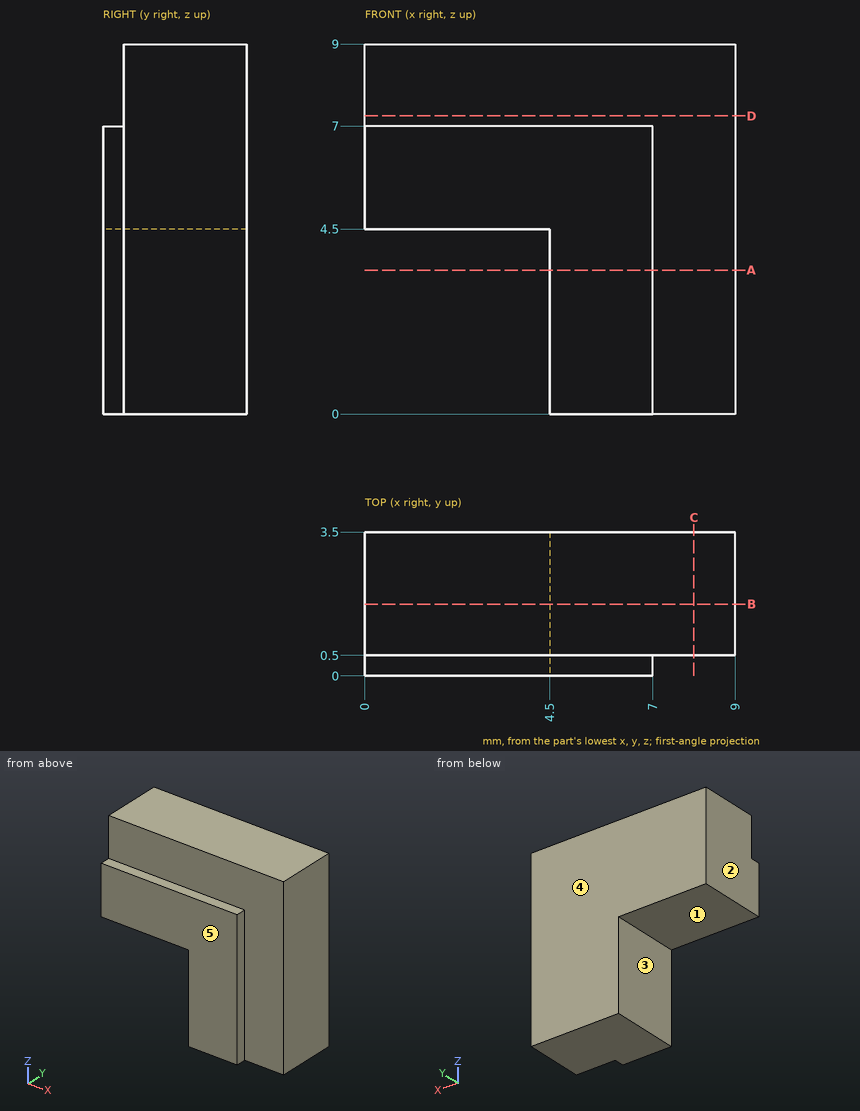
Design review of the part shown in the three views and the two pictorial views. Dimensions are in mm from the part's minimum x, y and z. A direction names the side the tool comes from. Give positions to 0.01 mm unless a question says otherwise; leave off trailing zeros. Write each loop counter-clockwise with the first axis right and the second up, starting at its lowest first coordinate (ties: lowest second). Pieces come first, ordered by that corner, then holes. Notation, with made-up numbers: M 72.5,31.5 L 85.5,31.5 A3 cw 85.5,36.5 Z; hole C 40.5,83.25 d10. An arc over 180 degrees is marked long. One line per question, with ' | ' between items. Start each with the question number.
Item 1: Wall thickness on line 1 (X direction, y = 0.4, z = 3.25); line 2 (Y direction, x = 7.75, z = 7); line 3 (Z direction, x = 3, y = 0.85): over which ranges is each line inside the solid? List them lowest first. Write a range as from..to.
Item 2: For pin 1 (1 mm diameter, centred on y = 1, z = 2.5, fed in from -X), flat-tipped, find the tip position at first contact; note if it passes through.
Item 3: We need section A-A on z = 3.5. Write out the cut boundary in (x, y), plus the area to 4 significant figures.
Item 4: We need section C-C on x = 8. Write out the cut boundary in (y, z).
Item 5: Draft analysis for pull direction Y (two halves, no side actions). For the marked faces 3, 4 and 5, state which applies: released by +Y, released by -Y, zero draft, split by the parting line, or undercut.
Item 6: We need section B-B on y = 1.75. Write out the cut boundary in (x, z).
Item 7: We need section D-D on z = 7.25. Write out the cut boundary in (x, y), plus the area to 3 significant figures.
Item 8: For the marked faces 1 and 2, list the 3-axis set-ups (+Z, -Z, +X, -X, +Y, -Y) from which the entire face can be reached by the end or side of a thin tool; tool diameter is ignored.
Results found:
1) line 1: x = 4.5..7 | line 2: y = 0.5..3.5 | line 3: z = 4.5..9
2) pin 1: stops at x = 4.5
3) outline: M 4.5,0 L 7,0 L 7,0.5 L 9,0.5 L 9,3.5 L 4.5,3.5 Z | area: 14.75 mm2
4) outline: M 0.5,0 L 3.5,0 L 3.5,9 L 0.5,9 Z
5) face 3: zero draft | face 4: released by +Y | face 5: released by -Y
6) outline: M 0,4.5 L 4.5,4.5 L 4.5,0 L 9,0 L 9,9 L 0,9 Z
7) outline: M 0,0.5 L 9,0.5 L 9,3.5 L 0,3.5 Z | area: 27.0 mm2
8) face 1: -Z, -X, +Y, -Y | face 2: +Z, -Z, -X, +Y, -Y
